```python
from build123d import *

# Parameters (mm, degrees)
T_LE_DE_BASE_PLI_E1_DEPTH = 10
ENL_V_MAT_EXTRU_1_REACH   = 32.256
ESQUISSE6_R               = 1.85
ENL_V_MAT_EXTRU_2_REACH   = 31.857


# Sheet-metal steps are written as plain solids
with BuildPart() as part:
    # Esquisse1 → Tôle de base pliée1 (new body)
    with BuildSketch(Plane.XY):
        with BuildLine():
            Line((0, 15), (0, 2.2))
            ThreePointArc((0, 2.2), (0.644365081, 0.644365081), (2.2, 0))
            Line((2.2, 0), (25, 0))
            Line((25, 0), (25, 1.2))
            Line((25, 1.2), (2.2, 1.2))
            ThreePointArc((2.2, 1.2), (1.492893219, 1.492893219), (1.2, 2.2))
            Line((1.2, 2.2), (1.2, 15))
            Line((1.2, 15), (0, 15))
        make_face()
    extrude(amount=T_LE_DE_BASE_PLI_E1_DEPTH)

    # Esquisse6 → Enlèv. mat.-Extru.1 (cut, up to next)
    with BuildSketch(Plane(origin=(0, 1.2, 0), x_dir=(1, 0, 0), z_dir=(0, 1, 0)), mode=Mode.PRIVATE) as enl_v_mat_extru_1_sk1:
        with Locations(Location((20, -5, 0), (0, 0, 270))):
            Circle(ESQUISSE6_R)
    enl_v_mat_extru_1_tool1 = extrude(enl_v_mat_extru_1_sk1.sketch, amount=-ENL_V_MAT_EXTRU_1_REACH, mode=Mode.PRIVATE) & part.part
    add(enl_v_mat_extru_1_tool1.solids().sort_by_distance((20, 1.2, 5))[0], mode=Mode.SUBTRACT)

    # Esquisse7 → Enlèv. mat.-Extru.2 (cut, up to next)
    with BuildSketch(Plane(origin=(1.2, 0, 0), x_dir=(0, 0, -1), z_dir=(1, 0, 0)), mode=Mode.PRIVATE) as enl_v_mat_extru_2_sk1:
        with BuildLine():
            Line((-3.15, 10), (-3.15, 7.2))
            ThreePointArc((-3.15, 7.2), (-5, 5.35), (-6.85, 7.2))
            Line((-6.85, 7.2), (-6.85, 10))
            ThreePointArc((-6.85, 10), (-5, 11.85), (-3.15, 10))
        make_face()
    enl_v_mat_extru_2_tool1 = extrude(enl_v_mat_extru_2_sk1.sketch, amount=-ENL_V_MAT_EXTRU_2_REACH, mode=Mode.PRIVATE) & part.part
    add(enl_v_mat_extru_2_tool1.solids().sort_by_distance((1.2, 8.6, 5))[0], mode=Mode.SUBTRACT)


solid = part.part
```
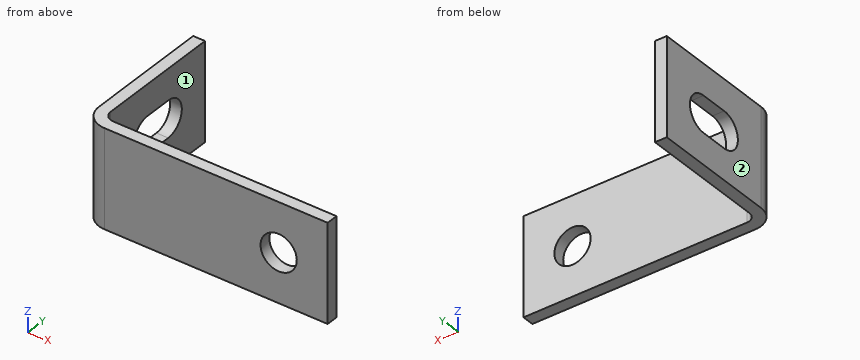
Part model, mm, in its own coordinate system. Face numbers are marked on the shaded views. A direction names the side the tool comes from. Give positions to 0.01 mm unless a question says otherwise; leave off trailing zeros. Order: outer loops, then holes, each group sorted by start corner. A loop starts at its lowest first (then second) coordinate and runs counter-clockwise, first axis right, second up. Notation, with made-up numbers: M -37,-9 L -1,-9 A19 cw -1,0 Z; hole C -21.5,50.5 d9. An arc over 180 degrees is marked long. Use a Markdown table: item, result. Add a question column.
(1) Probe line 1 along Y through (x, z) = (11.75, 1.25); line 2 along X through (y, z) = (0.6, 5). List the from-to ranges inside material, lowest first. Write a range as [from, to].
(2) 3-axis set-ups, long thin cutter, end or side, ignore diameter. For the marked faces 1 and 2: which of +Z, -Z, +X, -X, +Y, -Y reach the whole face in a straight line?
(3) Drop flat-ended pins along their axis: P1, Ø1.5, axis at x = 22, z = 1.5, coming from the +Y side; P2, Ø5, axis at x = 4, z = 7, coming from the +Y side. Give the stop position or say it passes through.
(4) Saw through at A-A, the plane x = 20. Give the cut face in (y, z).
(5) Saw through at D-D, the plane z = 2. Give the cut face in (x, y).
(6) Saw through at C-C, the plane z = 5. Give the cut face in (x, y), and give its area (3 significant figures).
Answer key:
| question | item | result |
|---|---|---|
| 1 | line 1 | [0, 1.2] |
| 1 | line 2 | [0.69, 18.15], [21.85, 25] |
| 2 | face 1 | +Z, -Z, +X, +Y |
| 2 | face 2 | +Z, -Z, -X, +Y, -Y |
| 3 | P1 | y = 1.2 |
| 3 | P2 | y = 1.49 |
| 4 | outline | M 0,0 L 1.2,0 L 1.2,3.15 L 0,3.15 Z; M 0,6.85 L 1.2,6.85 L 1.2,10 L 0,10 Z |
| 5 | outline | M 0,2.2 A2.2 ccw 2.2,0 L 25,0 L 25,1.2 L 2.2,1.2 A1 cw 1.2,2.2 L 1.2,15 L 0,15 Z |
| 6 | outline | M 0,2.2 A2.2 ccw 2.2,0 L 18.15,0 L 18.15,1.2 L 2.2,1.2 A1 cw 1.2,2.2 L 1.2,5.35 L 0,5.35 Z; M 0,11.85 L 1.2,11.85 L 1.2,15 L 0,15 Z; M 21.85,0 L 25,0 L 25,1.2 L 21.85,1.2 Z |
| 6 | area | 33.5 mm^2 |
